The figure shows three views and two pictorial views of one solid part (mm, origin at its lowest corner). Answer the questions. A direction names the side the tool comes from. Round coordinates to 2 decimals unless told otherwise and drop trailing zeros. Order: outer loops, then holes, each group sorted by start corner. A loop starts at its lowest first (then second) coordinate and runs counter-clockwise, first axis right, second up. Notation, with made-up numbers: (64, 19.5) - (120, 19.5) arc R15 cw to (120, 47.5) - close; hole circle Ø11 at (76.5, 28). An arc over 180 degrees is marked (long way). One line per item, written item: value. Start each with the question number.
1. Section C-C, the plane x = 8.65 is taken. Give the vertices of the cut face in (y, z).
2. A tool of negligible diameter and unlimited length cuts with its end or side. For the marked faces 4 and 5, from which of +Z, -Z, +X, -X, +Y, -Y can it reach the whole face along a straight path? Write none if from no direction.
3. Section A-A, the plane x = 11.65 is taken. Give the vertices of the cut face in (y, z), then the cut area to 3 significant figures.
4. Straight lines are drawn through the part: line 1 (X direction, y = 2.4, z = 11.5); line 2 (Y direction, x = 1.5, z = 2.75); line 3 (X direction, y = 10.5, z = 1.25). For each, find the intervals that lie inside material, in ascending order.
5. Section D-D, the plane z = 11.5 is taken. Give the vertices of the cut face in (x, y), then the cut area to 3 significant figures.
6. A flat-ended cylindrical pin translates along its axis: P1, Ø2, axis at x = 15.5, z = 10.5, coming from the +Y side. Find the tip coordinate at first contact, or state that the pin passes through.
7. For a pull along X with two mould halves and no side action, classify the marked faces 1, 2 and 3 as released by +X, released by -X, zero draft, split by the parting line, or undercut.
8. Section B-B, the plane y = 20 is taken. Give the vertices of the cut face in (x, z), then the cut area to 3 significant figures.
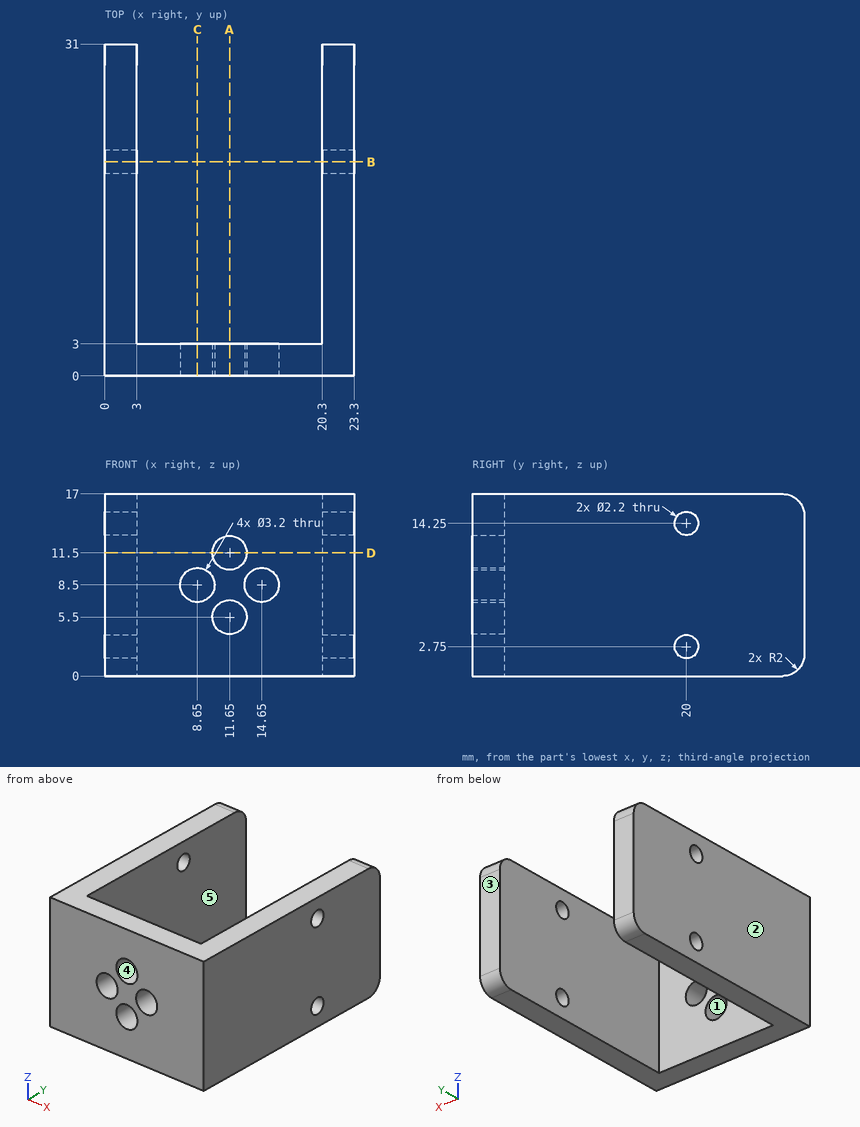
Answer list:
1. outline: (0, 0) - (3, 0) - (3, 6.9) - (0, 6.9) - close; (0, 10.1) - (3, 10.1) - (3, 17) - (0, 17) - close
2. face 4: +Y, -Y
2. face 5: +Z, -Z, +Y
3. outline: (0, 0) - (3, 0) - (3, 3.9) - (0, 3.9) - close; (0, 7.1) - (3, 7.1) - (3, 9.9) - (0, 9.9) - close; (0, 13.1) - (3, 13.1) - (3, 17) - (0, 17) - close
3. area: 31.8 mm²
4. line 1: x = 0 to 10.05, 13.25 to 23.3
4. line 2: y = 0 to 18.9, 21.1 to 31
4. line 3: x = 0 to 3, 20.3 to 23.3
5. outline: (0, 0) - (10.05, 0) - (10.05, 3) - (3, 3) - (3, 31) - (0, 31) - close; (13.25, 0) - (23.3, 0) - (23.3, 31) - (20.3, 31) - (20.3, 3) - (13.25, 3) - close
5. area: 228 mm²
6. P1: stops at y = 3
7. face 1: undercut
7. face 2: released by -X
7. face 3: zero draft
8. outline: (0, 0) - (3, 0) - (3, 1.65) - (0, 1.65) - close; (0, 3.85) - (3, 3.85) - (3, 13.15) - (0, 13.15) - close; (0, 15.35) - (3, 15.35) - (3, 17) - (0, 17) - close; (20.3, 0) - (23.3, 0) - (23.3, 1.65) - (20.3, 1.65) - close; (20.3, 3.85) - (23.3, 3.85) - (23.3, 13.15) - (20.3, 13.15) - close; (20.3, 15.35) - (23.3, 15.35) - (23.3, 17) - (20.3, 17) - close
8. area: 75.6 mm²
